```python
from build123d import *

# Parameters (mm, degrees)
SKETCH1_W               = 80
SKETCH1_H               = 60
BOSS_EXTRUDE1_DEPTH     = 2.5
CUT_EXTRUDE4_DEPTH      = 51.062460986
CUT_EXTRUDE4_DEPTH_BACK = 51.062460986
SKETCH2_R               = 1.6
SKETCH3_W               = 2.5
SKETCH3_H               = 20.5
BOSS_EXTRUDE2_DEPTH     = 66.5
SKETCH4_W               = 80
SKETCH4_H               = 5.5
BOSS_EXTRUDE3_DEPTH     = 2.5
SKETCH5_W               = 2.5
SKETCH5_H               = 5.5
BOSS_EXTRUDE4_DEPTH     = 66.5
SKETCH6_W               = 2.5
SKETCH6_H               = 5.5
CUT_EXTRUDE5_DEPTH      = 66.5
SKETCH9_W               = 2.5
SKETCH9_H               = 2.5
BOSS_EXTRUDE5_DEPTH     = 66.5
SKETCH11_R              = 4.75
CUT_EXTRUDE6_DEPTH      = 2.5
SKETCH15_W              = 2.5
SKETCH15_H              = 23
BOSS_EXTRUDE6_DEPTH     = 8
SKETCH17_W              = 2.5
SKETCH17_H              = 74.5
BOSS_EXTRUDE7_DEPTH     = 2
SKETCH18_R              = 1.6
CUT_EXTRUDE7_DEPTH      = 2.5
SKETCH21_W              = 80
SKETCH21_H              = 2.5
BOSS_EXTRUDE8_DEPTH     = 2
SKETCH22_W              = 4.25
SKETCH22_H              = 74.5
CUT_EXTRUDE8_DEPTH      = 2.5
FILLET1_R               = 5
SKETCH23_W              = 15.225
SKETCH23_H              = 67.5
BOSS_EXTRUDE10_DEPTH    = 2.5
SKETCH24_W              = 95.225
SKETCH24_H              = 10
CUT_EXTRUDE9_DEPTH      = 101.031498164
SKETCH26_W              = 2.5
SKETCH26_H              = 20.75
BOSS_EXTRUDE11_DEPTH    = 74.5
SKETCH27_R              = 1.6
CUT_EXTRUDE10_DEPTH     = 2.5
SKETCH28_W              = 2.5
SKETCH28_H              = 20.75
CUT_EXTRUDE11_DEPTH     = 74.5
SKETCH29_W              = 20.75
SKETCH29_H              = 19.625
CUT_EXTRUDE12_DEPTH     = 2.5
FILLET2_R               = 6
SKETCH31_W              = 13.325
SKETCH31_H              = 57.5
CUT_EXTRUDE13_DEPTH     = 2.5
SKETCH33_W              = 3
SKETCH33_H              = 57.5
CUT_EXTRUDE14_DEPTH     = 2.5
CUT_EXTRUDE15_DEPTH     = 2.5
SKETCH35_W              = 2.5
SKETCH35_H              = 20.75
CUT_EXTRUDE16_DEPTH     = 57.375


with BuildPart() as part:
    # Sketch1 → Boss-Extrude1 (new body)
    with BuildSketch(Plane(origin=(0, 0, 0), x_dir=(1, 0, 0), z_dir=(0, 1, 0))):
        Rectangle(SKETCH1_W, SKETCH1_H)
    extrude(amount=BOSS_EXTRUDE1_DEPTH)

    # Sketch2 → Cut-Extrude4 (cut, two sides: drawn at the far end of the back side and taken through both)
    with BuildSketch(Plane(origin=(0, 0, 0), x_dir=(1, 0, 0), z_dir=(0, 1, 0)).offset(-CUT_EXTRUDE4_DEPTH_BACK)):
        with BuildLine():
            Line((-6.25, -24), (-2.5, -24))
            ThreePointArc((-2.5, -24), (0, -21.5), (2.5, -24))
            Line((2.5, -24), (16.25, -24))
            Line((16.25, -24), (16.25, -18))
            Line((16.25, -18), (-6.25, -18))
            Line((-6.25, -18), (-6.25, -24))
        make_face()
        with BuildLine():
            Line((0, -26.5), (0, -30))
            Line((0, -30), (16.25, -30))
            Line((16.25, -30), (16.25, -24))
            Line((16.25, -24), (2.5, -24))
            ThreePointArc((2.5, -24), (1.767766953, -25.767766953), (0, -26.5))
        make_face()
        with BuildLine():
            ThreePointArc((-2.5, -24), (-1.767766953, -25.767766953), (0, -26.5))
            Line((0, -26.5), (0, -24))
            Line((0, -24), (-2.5, -24))
        make_face()
        with BuildLine():
            Line((0, -24), (0, -26.5))
            ThreePointArc((0, -26.5), (1.767766953, -25.767766953), (2.5, -24))
            Line((2.5, -24), (0, -24))
        make_face()
        with BuildLine():
            Line((-2.5, -24), (0, -24))
            Line((0, -24), (2.5, -24))
            ThreePointArc((2.5, -24), (0, -21.5), (-2.5, -24))
        make_face()
        with BuildLine():
            ThreePointArc((-2.5, -24), (-1.767766953, -25.767766953), (0, -26.5))
            Line((0, -26.5), (0, -24))
            Line((0, -24), (-2.5, -24))
        make_face()
        with BuildLine():
            Line((0, -24), (0, -26.5))
            ThreePointArc((0, -26.5), (1.767766953, -25.767766953), (2.5, -24))
            Line((2.5, -24), (0, -24))
        make_face()
        with BuildLine():
            Line((-6.25, -30), (0, -30))
            Line((0, -30), (0, -26.5))
            ThreePointArc((0, -26.5), (-1.767766953, -25.767766953), (-2.5, -24))
            Line((-2.5, -24), (-6.25, -24))
            Line((-6.25, -24), (-6.25, -30))
        make_face()
        with Locations(Location((-8.625, -24, 0), (0, 0, 270))):
            Circle(SKETCH2_R)
        with Locations(Location((18.625, -24, 0), (0, 0, 270))):
            Circle(SKETCH2_R)
    extrude(amount=CUT_EXTRUDE4_DEPTH + CUT_EXTRUDE4_DEPTH_BACK, mode=Mode.SUBTRACT)

    # Sketch3 → Boss-Extrude2 (add)
    with BuildSketch(Plane(origin=(0, 2.5, 0), x_dir=(1, 0, 0), z_dir=(0, 1, 0))):
        with Locations((-38.75, -19.75)):
            Rectangle(SKETCH3_W, SKETCH3_H)
    extrude(amount=BOSS_EXTRUDE2_DEPTH)

    # Sketch4 → Boss-Extrude3 (add)
    with BuildSketch(Plane(origin=(0, 2.5, 0), x_dir=(1, 0, 0), z_dir=(0, 1, 0))):
        with Locations((0, -32.75)):
            Rectangle(SKETCH4_W, SKETCH4_H)
    extrude(amount=-BOSS_EXTRUDE3_DEPTH)

    # Sketch5 → Boss-Extrude4 (add)
    with BuildSketch(Plane(origin=(0, 2.5, 0), x_dir=(1, 0, 0), z_dir=(0, 1, 0))):
        with Locations((-38.75, -32.75)):
            Rectangle(SKETCH5_W, SKETCH5_H)
    extrude(amount=BOSS_EXTRUDE4_DEPTH)

    # Sketch6 → Cut-Extrude5 (cut)
    with BuildSketch(Plane(origin=(0, 69, 0), x_dir=(1, 0, 0), z_dir=(0, 1, 0))):
        with Locations((-38.75, -12.25)):
            Rectangle(SKETCH6_W, SKETCH6_H)
    extrude(amount=-CUT_EXTRUDE5_DEPTH, mode=Mode.SUBTRACT)

    # Sketch9 → Boss-Extrude5 (add)
    with BuildSketch(Plane(origin=(0, 2.5, 0), x_dir=(1, 0, 0), z_dir=(0, 1, 0))):
        with Locations((-38.75, -13.75)):
            Rectangle(SKETCH9_W, SKETCH9_H)
    extrude(amount=BOSS_EXTRUDE5_DEPTH)

    # Sketch11 → Cut-Extrude6 (cut)
    with BuildSketch(Plane(origin=(-37.5, 0, 0), x_dir=(0, 0, -1), z_dir=(1, 0, 0))):
        with Locations((-24, 54)):
            Circle(SKETCH11_R)
    extrude(amount=-CUT_EXTRUDE6_DEPTH, mode=Mode.SUBTRACT)

    # Sketch15 → Boss-Extrude6 (add)
    with BuildSketch(Plane(origin=(0, 69, 0), x_dir=(1, 0, 0), z_dir=(0, 1, 0))):
        with Locations((-38.75, -24)):
            Rectangle(SKETCH15_W, SKETCH15_H)
    extrude(amount=BOSS_EXTRUDE6_DEPTH)

    # Sketch17 → Boss-Extrude7 (add)
    with BuildSketch(Plane.XY.offset(35.5)):
        with Locations((-38.75, 39.75)):
            Rectangle(SKETCH17_W, SKETCH17_H)
    extrude(amount=BOSS_EXTRUDE7_DEPTH)

    # Sketch18 → Cut-Extrude7 (cut)
    with BuildSketch(Plane.ZY.offset(40)):
        with Locations((32, 36.5)):
            Circle(SKETCH18_R)
        with Locations((32, 71.5)):
            Circle(SKETCH18_R)
    extrude(amount=-CUT_EXTRUDE7_DEPTH, mode=Mode.SUBTRACT)

    # Sketch21 → Boss-Extrude8 (add)
    with BuildSketch(Plane.XY.offset(35.5)):
        with Locations((0, 1.25)):
            Rectangle(SKETCH21_W, SKETCH21_H)
    extrude(amount=BOSS_EXTRUDE8_DEPTH)

    # Sketch22 → Cut-Extrude8 (cut)
    with BuildSketch(Plane(origin=(-37.5, 0, 0), x_dir=(0, 0, -1), z_dir=(1, 0, 0))):
        with Locations((-14.625, 39.75)):
            Rectangle(SKETCH22_W, SKETCH22_H)
    extrude(amount=-CUT_EXTRUDE8_DEPTH, mode=Mode.SUBTRACT)

    # Fillet1
    fillet1_edges = [part.edges().sort_by_distance(p)[0] for p in [
        (-38.75, 77, 37.5),
        (-38.75, 77, 16.75),
    ]]
    fillet(fillet1_edges, radius=FILLET1_R)

    # Sketch23 → Boss-Extrude10 (add)
    with BuildSketch(Plane(origin=(0, 2.5, 0), x_dir=(1, 0, 0), z_dir=(0, 1, 0))):
        with Locations((47.6125, -3.75)):
            Rectangle(SKETCH23_W, SKETCH23_H)
    extrude(amount=-BOSS_EXTRUDE10_DEPTH)

    # Sketch24 → Cut-Extrude9 (cut, through all)
    with BuildSketch(Plane(origin=(0, 2.5, 0), x_dir=(1, 0, 0), z_dir=(0, 1, 0))):
        with Locations((7.6125, 25)):
            Rectangle(SKETCH24_W, SKETCH24_H)
    extrude(amount=-CUT_EXTRUDE9_DEPTH, mode=Mode.SUBTRACT)

    # Sketch26 → Boss-Extrude11 (add)
    with BuildSketch(Plane(origin=(0, 2.5, 0), x_dir=(1, 0, 0), z_dir=(0, 1, 0))):
        with Locations((-25.425, -27.125)):
            Rectangle(SKETCH26_W, SKETCH26_H)
    extrude(amount=BOSS_EXTRUDE11_DEPTH)

    # Sketch27 → Cut-Extrude10 (cut)
    with BuildSketch(Plane(origin=(-24.175, 0, 0), x_dir=(0, 0, -1), z_dir=(1, 0, 0))):
        with BuildLine():
            ThreePointArc((-28.75, 36.275), (-27.358757211, 32.916242789), (-24, 31.525))
            Line((-24, 31.525), (-24, 36.275))
            Line((-24, 36.275), (-28.75, 36.275))
        make_face()
        with BuildLine():
            Line((-24, 36.275), (-24, 31.525))
            ThreePointArc((-24, 31.525), (-20.641242789, 32.916242789), (-19.25, 36.275))
            ThreePointArc((-19.25, 36.275), (-24, 41.025), (-28.75, 36.275))
            Line((-28.75, 36.275), (-24, 36.275))
        make_face()
        with BuildLine():
            ThreePointArc((-28.75, 36.275), (-27.358757211, 32.916242789), (-24, 31.525))
            Line((-24, 31.525), (-24, 36.275))
            Line((-24, 36.275), (-28.75, 36.275))
        make_face()
        with BuildLine():
            Line((-24, 36.275), (-24, 31.525))
            ThreePointArc((-24, 31.525), (-20.641242789, 32.916242789), (-19.25, 36.275))
            ThreePointArc((-19.25, 36.275), (-24, 41.025), (-28.75, 36.275))
            Line((-28.75, 36.275), (-24, 36.275))
        make_face()
        with Locations((-32, 18.775)):
            Circle(SKETCH27_R)
        with Locations((-32, 53.775)):
            Circle(SKETCH27_R)
    extrude(amount=-CUT_EXTRUDE10_DEPTH, mode=Mode.SUBTRACT)

    # Sketch28 → Cut-Extrude11 (cut)
    with BuildSketch(Plane(origin=(0, 77, 0), x_dir=(1, 0, 0), z_dir=(0, 1, 0))):
        with Locations((-38.75, -27.125)):
            Rectangle(SKETCH28_W, SKETCH28_H)
    extrude(amount=-CUT_EXTRUDE11_DEPTH, mode=Mode.SUBTRACT)

    # Sketch29 → Cut-Extrude12 (cut)
    with BuildSketch(Plane(origin=(-24.175, 0, 0), x_dir=(0, 0, -1), z_dir=(1, 0, 0))):
        with Locations((-27.125, 67.1875)):
            Rectangle(SKETCH29_W, SKETCH29_H)
    extrude(amount=-CUT_EXTRUDE12_DEPTH, mode=Mode.SUBTRACT)

    # Fillet2
    fillet2_edges = [part.edges().sort_by_distance(p)[0] for p in [
        (-25.425, 57.375, 37.5),
        (-25.425, 57.375, 16.75),
    ]]
    fillet(fillet2_edges, radius=FILLET2_R)

    # Sketch31 → Cut-Extrude13 (cut)
    with BuildSketch(Plane(origin=(0, 2.5, 0), x_dir=(1, 0, 0), z_dir=(0, 1, 0))):
        with Locations((-33.3375, -8.75)):
            Rectangle(SKETCH31_W, SKETCH31_H)
    extrude(amount=-CUT_EXTRUDE13_DEPTH, mode=Mode.SUBTRACT)

    # Sketch33 → Cut-Extrude14 (cut)
    with BuildSketch(Plane(origin=(0, 2.5, 0), x_dir=(1, 0, 0), z_dir=(0, 1, 0))):
        with Locations((53.725, -8.75)):
            Rectangle(SKETCH33_W, SKETCH33_H)
    extrude(amount=-CUT_EXTRUDE14_DEPTH, mode=Mode.SUBTRACT)

    # Sketch34 → Cut-Extrude15 (cut)
    with BuildSketch(Plane(origin=(0, 2.5, 0), x_dir=(1, 0, 0), z_dir=(0, 1, 0))):
        Polygon((-24.175, -24.625), (-24.175, -27.125), (-24.175, -29.625), (-19.175, -29.625), (-19.175, -24.625), align=None)
        Polygon((-19.175, -22.125), (-19.175, -24.625), (-19.175, -29.625), (-19.175, -32.125), (-16.675, -32.125), (-16.675, -22.125), align=None)
    extrude(amount=-CUT_EXTRUDE15_DEPTH, mode=Mode.SUBTRACT)

    # Sketch35 → Cut-Extrude16 (cut)
    with BuildSketch(Plane(origin=(0, 57.375, 0), x_dir=(1, 0, 0), z_dir=(0, 1, 0))):
        with Locations((-25.425, -27.125)):
            Rectangle(SKETCH35_W, SKETCH35_H)
    extrude(amount=-CUT_EXTRUDE16_DEPTH, mode=Mode.SUBTRACT)


solid = part.part
```
Verification items for the finished model (mm, model axes). A direction names the side the tool comes from. Round coordinates to 2 decimals unless told otherwise and drop trailing zeros. Write each loop counter-clockwise with the first axis right and the second up, starting at its lowest first coordinate (ties: lowest second). Pieces come first, ordered by that corner, then holes.
1. Section check B-B on y = 1.5. Enter the section's corners in (x, z) (3 decimals).
2. Scan lines: L1, parallel to X at y = 1.1, z = 24 (3 decimals); L2, parallel to Z at x = 7, y = 0.75; L3, parallel to X at y = 2.15, z = 19.5 (3 decimals). Record each from-to range of solid material in increasing order.
3. Access from +Z, -Z, +X, -X, +Y, -Y to the whole of each face (thin tool, end or side, straight path). Record for faces 1 (the flat face through (-19.175, 1, 31)), 2 (the flat face through (-24.175, 1, 34)), 3 (the flat face through (-22, 1, 24.625)), 4 (the flat face through (12, 0, 8)).
4. Gauge pin test, flat ends, axial feed: P1, Ø0.8, axis at y = 1, z = 29.5, coming from the -X side (3 decimals); P2, Ø3, axis at x = -8.625, z = 24, coming from the +Y side. Record the tip position at first contact, or that the pin passes through.
5. Draft check along Z on faces 5 (the flat face through (12, 1, -20)), 6 (the flat face through (16.25, 1, 24)), 7 (the flat face through (52.225, 1, 9)). Enter one of: +Z half, -Z half, draft (parallel to the pull), parting line (faces both ways), or undercut.
6. Section check A-A on z = 23.5. Enter the section's corners in (x, y) (3 decimals).
Answer:
1. outline: (-26.675, -20) - (52.225, -20) - (52.225, 37.5) - (-24.175, 37.5) - (-24.175, 29.625) - (-19.175, 29.625) - (-19.175, 32.125) - (-16.675, 32.125) - (-16.675, 22.125) - (-19.175, 22.125) - (-19.175, 24.625) - (-24.175, 24.625) - (-24.175, 16.75) - (-26.675, 16.75) - close; hole circle Ø3.2 at (-8.625, 24); hole (-6.25, 18) - (16.25, 18) - (16.25, 30) - (-6.25, 30) - close; hole circle Ø3.2 at (18.625, 24)
2. L1: x = -24.175 to -19.175, -16.675 to -10.225, -7.025 to -6.25, 16.25 to 17.025, 20.225 to 52.225
2. L2: z = -20 to 18, 30 to 37.5
2. L3: x = -24.175 to -6.25, 16.25 to 52.225
3. face 1: +Y, -Y
3. face 2: +Z, -X, +Y, -Y
3. face 3: -X, +Y, -Y
3. face 4: +Z, -Z, +X, -X, -Y
4. P1: stops at x = -24.175
4. P2: passes through
5. face 5: -Z half
5. face 6: undercut
5. face 7: draft
6. outline: (-24.175, 0) - (-19.175, 0) - (-19.175, 2.5) - (-24.175, 2.5) - close; (-16.675, 0) - (-10.145, 0) - (-10.145, 2.5) - (-16.675, 2.5) - close; (-7.105, 0) - (-6.25, 0) - (-6.25, 2.5) - (-7.105, 2.5) - close; (16.25, 0) - (17.105, 0) - (17.105, 2.5) - (16.25, 2.5) - close; (20.145, 0) - (52.225, 0) - (52.225, 2.5) - (20.145, 2.5) - close
